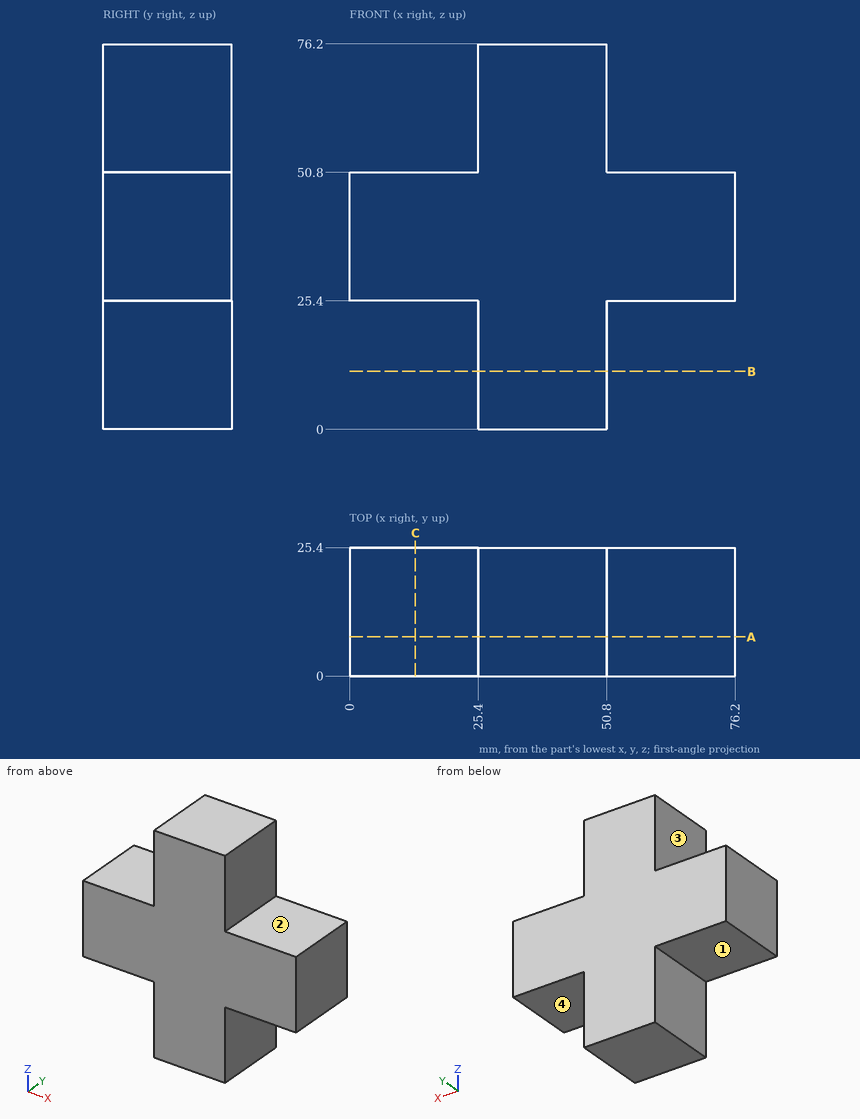
The drawing under review shows one solid part. Ordinate dimensions are in mm from its lowest x, y, z. A direction names the side the tool comes from. Round coordinates to 2 decimals unless told otherwise and drop trailing zeros. Loops run counter-clockwise (first coordinate to the right, second up) from the corner with the lowest first, then second, coordinate; pieces in that order, holes last. Notation, with made-up numbers: (29, 21.5) - (51, 21.5) arc R20 ccw to (51, 45.5) - close; hole circle Ø10 at (45, 1.5). An arc over 180 degrees is marked (long way). Use a Markdown table: item, result. Add a question column.
Q1. Machinability: for the marked faces 1, 2, 3 and 4, which of the approach directions +Z, -Z, +X, -X, +Y, -Y give a long, thin tool a straight path to every point of the face, cutting with its end or side? Answer none if there is none.
Q2. Add section C-C (x = 13). State the section outline as (y, z) points, plus the area to 3 significant figures.
Q3. Add section B-B (z = 11.5). State the section outline as (x, y) points, plus the area to 3 significant figures.
Q4. Insertion check: pin 1 Ø12.5 at (x, y) = (70, 19) entering from +Z; pin 2 Ø10 at (x, z) = (19, 58.5) entering from -Y; pin 3 Ø7.5 at (y, z) = (11.5, 58) entering from -X; pin 4 Ø7.5 at (y, z) = (11.5, 9) entering from +X. Each pin has a flat end and moves straight along its axis. Give the tip position at first contact, or say it passes through.
Q5. For probe 1 along Z at (x, y) = (6, 13.5), list the stretches that pass through material, from the lowest coordinate up.
Q6. Add section A-A (y = 7.75). State the section outline as (x, z) points, plus the area to 3 significant figures.
Worked answers:
| question | item | result |
|---|---|---|
| 1 | face 1 | -Z, -X, +Y, -Y |
| 1 | face 2 | +Z, +X, +Y, -Y |
| 1 | face 3 | +Z, -X, +Y, -Y |
| 1 | face 4 | -Z, +X, +Y, -Y |
| 2 | outline | (0, 25.4) - (25.4, 25.4) - (25.4, 50.8) - (0, 50.8) - close |
| 2 | area | 645 mm² |
| 3 | outline | (25.4, 0) - (50.8, 0) - (50.8, 25.4) - (25.4, 25.4) - close |
| 3 | area | 645 mm² |
| 4 | pin 1 | z = 50.8 |
| 4 | pin 2 | through |
| 4 | pin 3 | x = 25.4 |
| 4 | pin 4 | x = 50.8 |
| 5 | probe 1 | 25.4 to 50.8 |
| 6 | outline | (0, 25.4) - (25.4, 25.4) - (25.4, 0) - (50.8, 0) - (50.8, 25.4) - (76.2, 25.4) - (76.2, 50.8) - (50.8, 50.8) - (50.8, 76.2) - (25.4, 76.2) - (25.4, 50.8) - (0, 50.8) - close |
| 6 | area | 3,230 mm² |
